```python
from build123d import *

# Parameters (mm, degrees)
F0_R     = 11.9647327703
F1_DEPTH = 36.7
F2_R     = 6.0094743431
F3_DEPTH = 36.701


# Not quite as in the source:
# - a fillet or chamfer that OpenCascade refuses, or shapes differently, is made with other operations: its cross-section is extruded or revolved along the edge and cut away or added


with BuildPart() as f1:
    # F0 (on Top) → F1 (new body)
    with BuildSketch(Plane.XY):
        Circle(F0_R)
    extrude(amount=F1_DEPTH)

    # F2 (on face) → F3 (cut, through all)
    with BuildSketch(Plane.XY.offset(36.7)):
        with Locations((-1.6841825563, 1.5192364808)):
            Circle(F2_R)
    extrude(amount=-F3_DEPTH, mode=Mode.SUBTRACT)

    # F4: fillet of radius 5 on 1 edges, made by hand

    # F4_s1 → F4_t2 (revolve, cut)
    with BuildSketch(Plane.XZ):
        with BuildLine():
            ThreePointArc((11.9647327703, 31.7), (10.5002666762, 35.2355339059), (6.9647327703, 36.7))
            Line((6.9647327703, 36.7), (11.9647327703, 36.7))
            Line((11.9647327703, 36.7), (11.9647327703, 31.7))
        make_face()
    revolve(axis=Axis((0, 0, 36.7), (0, 0, 1)), mode=Mode.SUBTRACT)


solid = f1.part
```
The listing builds one solid part. Answer for the finished solid, in the listing's coordinates (mm). Give positions to 0.01 mm unless a question says otherwise; leave off trailing zeros. Write each loop counter-clockwise with the first axis right and the second up, starting at its lowest first coordinate (ties: lowest second). Pieces come first, ordered by that corner, then holes. Notation, with made-up numbers: (-15.75, 45) - (4.25, 45) arc R12 cw to (4.25, 60) - close; hole circle Ø10 at (-5.5, -20). An arc over 180 degrees is marked (long way). Use one line per item in the form item = value. Start each with the question number.
1) Consider line 1 along X through (y, z) = (1.5, 5); line 2 along Y through (x, z) = (-6.5, 25); line 3 along Y through (x, z) = (-3.5, 15). Determine where each line is inside the solid, lowest interval first. Write a range as from..to.
2) The mould has two halves that part along Y. Classify faces 1 (the face through (-2.987, -4.347, 18.607)), 2 (the face through (5, 0, 0)), 3 (the face through (-2.59, -11.68, 15.63)): pulls with the +Y half, pulls with the -Y half, needs draft (parallel to the pull), parting line crosses it, or undercut.
3) Flat-ended cylindrical pins translate along their axes: pin 1 Ø10 at (x, z) = (9.5, 29) entering from +Y; pin 2 Ø5 at (x, z) = (3, 9) entering from -Y; pin 3 Ø7 at (x, y) = (-1.68, 1.52) entering from +Z; pin 4 Ø2 at (y, z) = (3, 21) entering from -X. Find the tip coordinate at first contact, or state that the pin passes through.
4) Find section A-A on y = 0. Determine the outline of the cut face in (x, z), plus the area to 3 significant figures.
5) Find section C-C on z = 30.5. Determine the outline of the cut face in (x, y).
6) Find section B-B on x = 0. Determine the outline of the cut face in (y, z), plus the area to 3 significant figures.
Geometry results:
q1.line_1 = -11.87..-7.69, 4.33..11.87
q1.line_2 = -10.05..-2.08, 5.11..10.05
q1.line_3 = -11.44..-4.21, 7.25..11.44
q2.face_1 = undercut
q2.face_2 = needs draft
q2.face_3 = parting line crosses it
q3.pin_1 = 11.09
q3.pin_2 = -11.95
q3.pin_3 = through
q3.pin_4 = -11.8
q4.outline = (-11.96, 0) - (-7.5, 0) - (-7.5, 36.67) arc R5 ccw to (-11.96, 31.7) - close; (4.13, 0) - (11.96, 0) - (11.96, 31.7) arc R5 ccw to (6.96, 36.7) - (4.13, 36.7) - close
q4.area = 441 mm2
q5.outline = circle Ø23.93 at (0, 0); hole circle Ø12.02 at (-1.68, 1.52)
q6.outline = (-11.96, 0) - (-4.25, 0) - (-4.25, 36.7) - (-6.96, 36.7) arc R5 ccw to (-11.96, 31.7) - close; (7.29, 0) - (11.96, 0) - (11.96, 31.7) arc R5 ccw to (7.29, 36.69) - close
q6.area = 444 mm2
